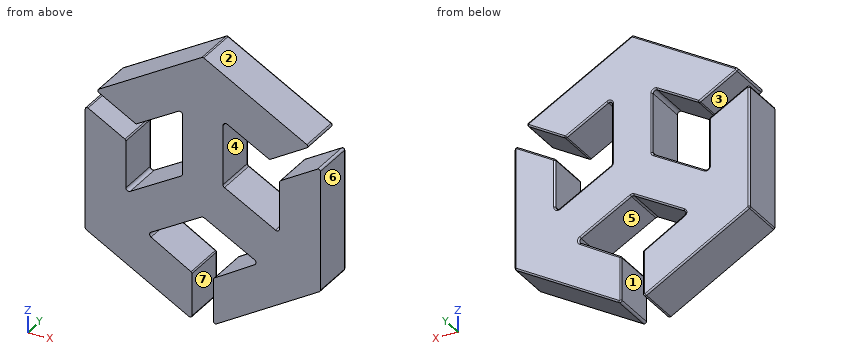
```python
from build123d import *

# Parameters (mm, degrees)
BOSS_EXTRUDE1_DEPTH = 12
FILLET1_R           = 0.4


with BuildPart() as part:
    # Sketch2 → Boss-Extrude1 (new body)
    with BuildSketch(Plane(origin=(0, 0, 0), x_dir=(1, 0, 0), z_dir=(0, 1, 0))):
        with BuildLine():
            Line((30.685392159, 42.367399762), (17.394899403, 49.906124645))
            ThreePointArc((17.394899403, 49.906124645), (17.014988006, 50.549604576), (17.379556544, 51.201899657))
            Line((17.379556544, 51.201899657), (27.955799295, 57.536628388))
            ThreePointArc((27.955799295, 57.536628388), (28.133885568, 57.719055755), (28.198880034, 57.96557185))
            Line((28.198880034, 57.96557185), (28.198880034, 69.110408185))
            ThreePointArc((28.198880034, 69.110408185), (27.948584386, 69.543591445), (27.448289088, 69.543079166))
            Line((27.448289088, 69.543079166), (0.249409054, 53.790247635))
            ThreePointArc((0.249409054, 53.790247635), (0.06681674, 53.607281006), (0, 53.357576654))
            Line((0, 53.357576654), (0, 21.946144977))
            ThreePointArc((0, 21.946144977), (0.250295648, 21.512961717), (0.750590946, 21.513473996))
            Line((0.750590946, 21.513473996), (10.485126092, 27.151444824))
            ThreePointArc((10.485126092, 27.151444824), (10.667718406, 27.334411453), (10.734535146, 27.584115805))
            Line((10.734535146, 27.584115805), (10.734535146, 39.938347903))
            ThreePointArc((10.734535146, 39.938347903), (11.107061322, 40.586432398), (11.854571179, 40.590707723))
            Line((11.854571179, 40.590707723), (25.329101543, 32.94759176))
            ThreePointArc((25.329101543, 32.94759176), (25.607150005, 32.672705765), (25.70906551, 32.29523194))
            Line((25.70906551, 32.29523194), (25.70906551, 16.68056549))
            ThreePointArc((25.70906551, 16.68056549), (25.336539334, 16.032480996), (24.589029478, 16.02820567))
            Line((24.589029478, 16.02820567), (13.662855507, 22.22582536))
            ThreePointArc((13.662855507, 22.22582536), (13.413917055, 22.29091376), (13.165573873, 22.223589794))
            Line((13.165573873, 22.223589794), (3.560555046, 16.6606312))
            ThreePointArc((3.560555046, 16.6606312), (3.311146766, 16.227080269), (3.562079511, 15.79440989))
            Line((3.562079511, 15.79440989), (30.80636171, 0.143083992))
            ThreePointArc((30.80636171, 0.143083992), (31.055428191, 0.076634322), (31.304494672, 0.143083992))
            Line((31.304494672, 0.143083992), (58.548776872, 15.79440989))
            ThreePointArc((58.548776872, 15.79440989), (58.799709616, 16.227080269), (58.550301337, 16.6606312))
            Line((58.550301337, 16.6606312), (48.94528251, 22.223589794))
            ThreePointArc((48.94528251, 22.223589794), (48.696939328, 22.29091376), (48.448000876, 22.22582536))
            Line((48.448000876, 22.22582536), (37.521826905, 16.02820567))
            ThreePointArc((37.521826905, 16.02820567), (36.774317049, 16.032480996), (36.401790873, 16.68056549))
            Line((36.401790873, 16.68056549), (36.401790873, 32.29523194))
            ThreePointArc((36.401790873, 32.29523194), (36.503706378, 32.672705765), (36.78175484, 32.94759176))
            Line((36.78175484, 32.94759176), (50.256285204, 40.590707723))
            ThreePointArc((50.256285204, 40.590707723), (51.003795061, 40.586432398), (51.376321236, 39.938347903))
            Line((51.376321236, 39.938347903), (51.376321236, 27.584115805))
            ThreePointArc((51.376321236, 27.584115805), (51.443137977, 27.334411453), (51.625730291, 27.151444824))
            Line((51.625730291, 27.151444824), (61.360265437, 21.513473996))
            ThreePointArc((61.360265437, 21.513473996), (61.860560735, 21.512961717), (62.110856383, 21.946144977))
            Line((62.110856383, 21.946144977), (62.110856383, 53.357576654))
            ThreePointArc((62.110856383, 53.357576654), (62.044039643, 53.607281006), (61.861447329, 53.790247635))
            Line((61.861447329, 53.790247635), (34.662567295, 69.543079166))
            ThreePointArc((34.662567295, 69.543079166), (34.162271997, 69.543591445), (33.911976349, 69.110408185))
            Line((33.911976349, 69.110408185), (33.911976349, 57.96557185))
            ThreePointArc((33.911976349, 57.96557185), (33.976970814, 57.719055755), (34.155057088, 57.536628388))
            Line((34.155057088, 57.536628388), (44.731299839, 51.201899657))
            ThreePointArc((44.731299839, 51.201899657), (45.095868377, 50.549604576), (44.71595698, 49.906124645))
            Line((44.71595698, 49.906124645), (31.425464224, 42.367399762))
            ThreePointArc((31.425464224, 42.367399762), (31.055428191, 42.269759582), (30.685392159, 42.367399762))
        make_face()
    extrude(amount=BOSS_EXTRUDE1_DEPTH)

    # Fillet1
    fillet1_edges = [part.edges().sort_by_distance(p)[0] for p in [
        (31.055428191, 12, -0.076634322),
        (44.926635772, 12, -7.968746941),
        (58.799709616, 12, -16.227080269),
        (53.747791923, 12, -19.442110497),
        (48.696939328, 12, -22.29091376),
        (42.98491389, 12, -19.127015515),
        (36.774317049, 12, -16.032480996),
        (36.401790873, 12, -24.487898715),
        (17.014988006, 12, -50.549604576),
        (36.503706378, 12, -32.672705765),
        (43.519020022, 12, -36.769149742),
        (51.003795061, 12, -40.586432398),
        (51.376321236, 12, -33.761231854),
        (51.443137977, 12, -27.334411453),
        (56.492997864, 12, -24.33245941),
        (61.860560735, 12, -21.512961717),
        (62.110856383, 12, -37.651860815),
        (62.044039643, 12, -53.607281006),
        (48.262007312, 12, -61.666663401),
        (22.667677919, 12, -54.369264023),
        (34.162271997, 12, -69.543591445),
        (33.911976349, 12, -63.537990018),
        (33.976970814, 12, -57.719055755),
        (39.443178463, 12, -54.369264023),
        (45.095868377, 12, -50.549604576),
        (38.070710602, 12, -46.136762203),
        (28.133885568, 12, -57.719055755),
        (28.198880034, 12, -63.537990018),
        (27.948584386, 12, -69.543591445),
        (13.848849071, 12, -61.666663401),
        (0.06681674, 12, -53.607281006),
        (0, 12, -37.651860815),
        (0.250295648, 12, -21.512961717),
        (5.617858519, 12, -24.33245941),
        (31.055428191, 12, -42.269759582),
        (10.667718406, 12, -27.334411453),
        (10.734535146, 12, -33.761231854),
        (11.107061322, 12, -40.586432398),
        (18.591836361, 12, -36.769149742),
        (25.607150005, 12, -32.672705765),
        (25.70906551, 12, -24.487898715),
        (25.336539334, 12, -16.032480996),
        (19.125942492, 12, -19.127015515),
        (13.413917055, 12, -22.29091376),
        (8.36306446, 12, -19.442110497),
        (24.040145781, 12, -46.136762203),
        (3.311146766, 12, -16.227080269),
        (17.184220611, 12, -7.968746941),
    ]]
    fillet(fillet1_edges, radius=FILLET1_R)


solid = part.part
```
For this review, take the finished solid that the model builds, in its own axes (mm). Face numbers are marked on the shaded views. A direction names the side the tool comes from. Give positions to 0.01 mm unless a question says otherwise; leave off trailing zeros.
1) The part is to be moulded in two halves that separate along Z. For the marked faces 1, 2, 3 and 4, say which applies: released by +Z, released by -Z, zero draft, split by the parting line, or undercut.
2) Wall thickness on line 1 (Z direction, x = 38, y = 5); line 2 (X direction, y = 6.25, z = -44); line 3 (X direction, y = 0.75, z = -39): over which ranges is each line inside the solid? List them lowest first.
3) For the marked faces 5, 6 and 7, list the 3-axis set-ups (+Z, -Z, +X, -X, +Y, -Y) from which the entire face can be reached by the end or side of a thin tool; tool diameter is ignored.
4) Insertion check: pin 1 (5 mm diameter, centred on y = 10, z = -57.5, fed in from -X); pin 2 (1 mm diameter, centred on x = 48.5, y = 5.5, fed in from -Z); pin 3 (5 mm diameter, centred on x = 55, y = 7, fed in from +Z); pin 4 (6 mm diameter, centred on x = 21, z = -37.5, fed in from -Y). Each pin has a flat end and moves straight along its axis. Give the tip position at first contact, or say it passes through.
5) Take a section at A-A (x = 39). State how many separate pieces and enclosed holes the cut face has, then the cut area to 3 significant figures.
Derived:
1. face 1: zero draft
1. face 2: released by +Z
1. face 3: undercut
1. face 4: undercut
2. line 1: z = -67.61 to -55.23, -46.1 to -33.64, -16.3 to -3.99
2. line 2: x = 0 to 27.81, 34.3 to 62.11
2. line 3: x = 0 to 10.73, 14.66 to 47.45, 51.38 to 62.11
3. face 5: +Y, -Y
3. face 6: +Z, -Z, +X, +Y, -Y
3. face 7: -Z, +Y, -Y
4. pin 1: stops at x = 2.34
4. pin 2: stops at z = -61.82
4. pin 3: stops at z = -12.32
4. pin 4: stops at y = 0
5. separate pieces: 3
5. enclosed holes: 0
5. area: 446 mm2
